The model under review builds one solid part; all positions refer to its coordinate system, in mm. A direction names the side the tool comes from. Give positions to 0.01 mm unless a question says otherwise; leave off trailing zeros. Loops run counter-clockwise (first coordinate to the right, second up) from the corner with the lowest first, then second, coordinate; pieces in that order, holes last. Notation, with made-up numbers: M 47.25,-26.5 L 57.25,-26.5 A12 cw 57.25,-16.5 Z; hole C 80,70.25 d10. An arc over 180 degrees is marked long. Put each result on its own line as item: value. Start each with the question number.
```python
from build123d import *

# Parameters (mm, degrees)
SKETCH1_W           = 144
SKETCH1_H           = 80
BOSS_EXTRUDE1_DEPTH = 50
CUT_EXTRUDE1_REACH  = 98.354
SKETCH2_R           = 10
SKETCH2_R_2         = 13
CUT_EXTRUDE3_REACH  = 98.354
SKETCH3_W           = 144
SKETCH3_H           = 20
CUT_EXTRUDE4_REACH  = 108.226
SKETCH5_R           = 3
FILLET1_R           = 10
FILLET2_R           = 10
FILLET3_R           = 10
FILLET4_R           = 10
SKETCH6_R           = 5.5
CUT_EXTRUDE5_DEPTH  = 5


with BuildPart() as part:
    # Sketch1 → Boss-Extrude1 (new body)
    with BuildSketch(Plane.XY):
        Rectangle(SKETCH1_W, SKETCH1_H)
    extrude(amount=BOSS_EXTRUDE1_DEPTH)

    # Sketch2 → Cut-Extrude1 (cut, up to next)
    with BuildSketch(Plane.XY.offset(50), mode=Mode.PRIVATE) as cut_extrude1_sk1:
        Circle(SKETCH2_R)
    cut_extrude1_tool1 = extrude(cut_extrude1_sk1.sketch, amount=-CUT_EXTRUDE1_REACH, mode=Mode.PRIVATE) & part.part
    # Sketch2 → Cut-Extrude1 (cut, up to next)
    with BuildSketch(Plane.XY.offset(50), mode=Mode.PRIVATE) as cut_extrude1_sk2:
        with Locations((-50, 0)):
            Circle(SKETCH2_R_2)
    cut_extrude1_tool2 = extrude(cut_extrude1_sk2.sketch, amount=-CUT_EXTRUDE1_REACH, mode=Mode.PRIVATE) & part.part
    # Sketch2 → Cut-Extrude1 (cut, up to next)
    with BuildSketch(Plane.XY.offset(50), mode=Mode.PRIVATE) as cut_extrude1_sk3:
        with Locations(Location((50, 0, 0), (0, 0, 180))):
            Circle(SKETCH2_R_2)
    cut_extrude1_tool3 = extrude(cut_extrude1_sk3.sketch, amount=-CUT_EXTRUDE1_REACH, mode=Mode.PRIVATE) & part.part
    add(cut_extrude1_tool1.solids().sort_by_distance((0, 0, 50))[0], mode=Mode.SUBTRACT)
    add(cut_extrude1_tool2.solids().sort_by_distance((-50, 0, 50))[0], mode=Mode.SUBTRACT)
    add(cut_extrude1_tool3.solids().sort_by_distance((50, 0, 50))[0], mode=Mode.SUBTRACT)

    # Sketch3 → Cut-Extrude3 (cut, up to next)
    with BuildSketch(Plane.XY.offset(50), mode=Mode.PRIVATE) as cut_extrude3_sk1:
        with Locations((0, -30)):
            Rectangle(SKETCH3_W, SKETCH3_H)
    cut_extrude3_tool1 = extrude(cut_extrude3_sk1.sketch, amount=-CUT_EXTRUDE3_REACH, mode=Mode.PRIVATE) & part.part
    add(cut_extrude3_tool1.solids().sort_by_distance((0, -30, 50))[0], mode=Mode.SUBTRACT)

    # Sketch5 → Cut-Extrude4 (cut, up to next)
    with BuildSketch(Plane.XZ.offset(20), mode=Mode.PRIVATE) as cut_extrude4_sk1:
        with Locations(Location((-22, 34, 0), (0, 0, 270))):
            Circle(SKETCH5_R)
    cut_extrude4_tool1 = extrude(cut_extrude4_sk1.sketch, amount=-CUT_EXTRUDE4_REACH, mode=Mode.PRIVATE) & part.part
    # Sketch5 → Cut-Extrude4 (cut, up to next)
    with BuildSketch(Plane.XZ.offset(20), mode=Mode.PRIVATE) as cut_extrude4_sk2:
        with Locations(Location((-22, 14, 0), (0, 0, 270))):
            Circle(SKETCH5_R)
    cut_extrude4_tool2 = extrude(cut_extrude4_sk2.sketch, amount=-CUT_EXTRUDE4_REACH, mode=Mode.PRIVATE) & part.part
    add(cut_extrude4_tool1.solids().sort_by_distance((-22, -20, 34))[0], mode=Mode.SUBTRACT)
    add(cut_extrude4_tool2.solids().sort_by_distance((-22, -20, 14))[0], mode=Mode.SUBTRACT)

    # Fillet1
    fillet1_edges = [part.edges().sort_by_distance(p)[0] for p in [
        (72, -20, 25),
    ]]
    fillet(fillet1_edges, radius=FILLET1_R)

    # Fillet2
    fillet2_edges = [part.edges().sort_by_distance(p)[0] for p in [
        (72, 40, 25),
    ]]
    fillet(fillet2_edges, radius=FILLET2_R)

    # Fillet3
    fillet3_edges = [part.edges().sort_by_distance(p)[0] for p in [
        (-72, 40, 25),
    ]]
    fillet(fillet3_edges, radius=FILLET3_R)

    # Fillet4
    fillet4_edges = [part.edges().sort_by_distance(p)[0] for p in [
        (-72, -20, 25),
    ]]
    fillet(fillet4_edges, radius=FILLET4_R)

    # Sketch6 → Cut-Extrude5 (cut)
    with BuildSketch(Plane(origin=(0, 40, 0), x_dir=(1, 0, 0), z_dir=(0, 1, 0))):
        with Locations(Location((-22, -14, 0), (0, 0, 270))):
            Circle(SKETCH6_R)
        with Locations(Location((-22, -34, 0), (0, 0, 270))):
            Circle(SKETCH6_R)
    extrude(amount=-CUT_EXTRUDE5_DEPTH, mode=Mode.SUBTRACT)


solid = part.part
```
Item 1: Tool access review of faces 4 (the cylindrical face through (62.987, -0.572, 25.35)), 5 (the flat face through (-24.4, 35, 16.4)): name each direction out of +Z, -Z, +X, -X, +Y, -Y from which nothing blocks a thin tool from reaching the whole face with its end or side.
Item 2: Consider section C-C, the plane x = -22. Write out the cut boundary in (y, z).
Item 3: Draft analysis for pull direction Y (two halves, no side actions). For faces 1 (the cylindrical face through (-2.17, -9.76, 25.35)), 2 (the flat face through (-1, 10.4, 50)), 3 (the cylindrical face through (-69.15, -16.99, 24.65)), state which applies: +Y half, -Y half, draft (parallel to the pull), parting line (faces both ways), or undercut.
Item 4: Consider section A-A, the plane x = -50. Write out the cut boundary in (y, z).
Item 5: Clearance check with flat-ended pins moving along their axes: pin 1 Ø3.5 at (x, z) = (-22.5, 35) entering from +Y; pin 2 Ø9.5 at (x, z) = (-22, 14) entering from +Y; pin 3 Ø5 at (y, z) = (34, 11) entering from +X. State where each tip first meets the part, or that it passes through.
Item 6: Consider section D-D, the plane z = 6.5. Write out the cut boundary in (x, y).
Item 7: Consider section B-B, the plane z = 35. Write out the cut boundary in (x, y).
Item 8: To check wall thickness, follow L1, parallel to X at y = -0.5, z = 20; L2, parallel to X at y = -3, z = 7.5; L3, parallel to X at y = -11, z = 43. State the ranges of each line that lie inside material, in increasing order. Write a range as [from, to].
Report:
1. face 4: +Z, -Z
1. face 5: +Y
2. outline: M -20,0 L 40,0 L 40,8.5 L 35,8.5 L 35,11 L -20,11 Z; M -20,17 L 35,17 L 35,19.5 L 40,19.5 L 40,28.5 L 35,28.5 L 35,31 L -20,31 Z; M -20,37 L 35,37 L 35,39.5 L 40,39.5 L 40,50 L -20,50 Z
3. face 1: undercut
3. face 2: draft
3. face 3: -Y half
4. outline: M -20,0 L -13,0 L -13,50 L -20,50 Z; M 13,0 L 40,0 L 40,50 L 13,50 Z
5. pin 1: through
5. pin 2: y = 35
5. pin 3: x = 71.89
6. outline: M -72,-10 A10 ccw -62,-20 L 62,-20 A10 ccw 72,-10 L 72,30 A10 ccw 62,40 L -62,40 A10 ccw -72,30 Z; hole C -50,0 d26; hole C 0,0 d20; hole C 50,0 d26
7. outline: M -72,-10 A10 ccw -62,-20 L -24.83,-20 L -24.83,35 L -27.41,35 L -27.41,40 L -62,40 A10 ccw -72,30 Z; M -19.17,-20 L 62,-20 A10 ccw 72,-10 L 72,30 A10 ccw 62,40 L -16.59,40 L -16.59,35 L -19.17,35 Z; hole C -50,0 d26; hole C 0,0 d20; hole C 50,0 d26
8. L1: [-72, -62.99], [-37.01, -9.99], [9.99, 37.01], [62.99, 72]
8. L2: [-72, -62.65], [-37.35, -9.54], [9.54, 37.35], [62.65, 72]
8. L3: [-71.95, -56.93], [-43.07, 43.07], [56.93, 71.95]
